Work out the finished part from the listing and answer in its coordinate system (mm). Face numbers are marked on the shaded views. A direction names the side the tool comes from. Coordinates: 2 decimals unless noted, no trailing zeros. Order: outer loops, then holes, each group sorted by start corner. A loop starts at its lowest first (then second) coordinate and runs counter-clockwise, first axis right, second up. Notation, with made-up numbers: M -12,88.5 L 42,88.5 A21 cw 42,93.5 Z; hole C -2,-12 d3. An arc over 180 degrees is marked long. Use a Markdown table: item, result.
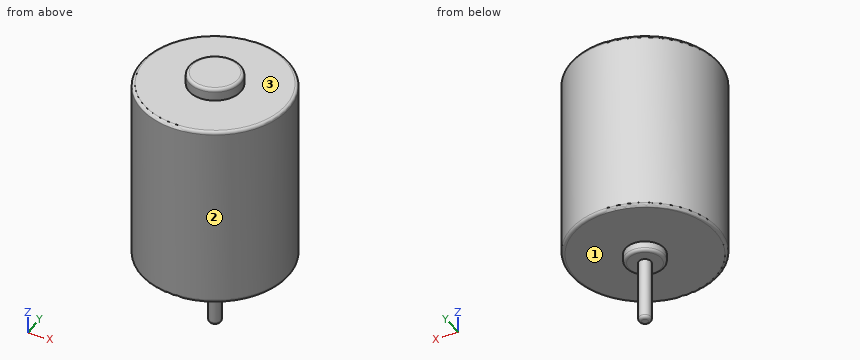
from build123d import *

# Parameters (mm, degrees)
SKETCH1_R           = 12.1
SKETCH1_R_2         = 3.175
SKETCH1_R_3         = 1
BOSS_EXTRUDE1_DEPTH = 30.5
SKETCH1_3_R         = 1
BOSS_EXTRUDE2_DEPTH = 12
SKETCH1_4_R         = 3.175
SKETCH1_4_R_2       = 1
BOSS_EXTRUDE3_DEPTH = 1.6
SKETCH2_R           = 4.25
BOSS_EXTRUDE4_DEPTH = 2
FILLET1_R           = 0.5


with BuildPart() as part:
    # Sketch1 → Boss-Extrude1 (new body)
    # profile 1 of 3: a face of its own
    with BuildSketch(Plane.XY):
        with Locations(Location((0, 0, 0), (0, 0, 180))):
            Circle(SKETCH1_R)
        Circle(SKETCH1_R_2, mode=Mode.SUBTRACT)
    # profile 2 of 3: a face of its own
    with BuildSketch(Plane.XY):
        Circle(SKETCH1_R_2)
        Circle(SKETCH1_R_3, mode=Mode.SUBTRACT)
    # profile 3 of 3: a face of its own
    with BuildSketch(Plane.XY):
        Circle(SKETCH1_R_3)
    extrude(amount=BOSS_EXTRUDE1_DEPTH)

    # Sketch1_3 → Boss-Extrude2 (add)
    with BuildSketch(Plane.XY):
        Circle(SKETCH1_3_R)
    extrude(amount=-BOSS_EXTRUDE2_DEPTH)

    # Sketch1_4 → Boss-Extrude3 (add)
    with BuildSketch(Plane.XY):
        Circle(SKETCH1_4_R)
        Circle(SKETCH1_4_R_2, mode=Mode.SUBTRACT)
    extrude(amount=-BOSS_EXTRUDE3_DEPTH)

    # Sketch2 → Boss-Extrude4 (add)
    with BuildSketch(Plane.XY.offset(30.5)):
        Circle(SKETCH2_R)
    extrude(amount=BOSS_EXTRUDE4_DEPTH)

    # Fillet1
    fillet1_edges = [part.edges().sort_by_distance(p)[0] for p in [
        (-3.175, 0, -1.6),
        (-4.25, 0, 32.5),
        (12.1, 0, 0),
        (12.1, 0, 30.5),
        (-1, 0, -12),
    ]]
    fillet(fillet1_edges, radius=FILLET1_R)


solid = part.part
1. For the marked faces 1, 2 and 3, determine the directions among +Z, -Z, +X, -X, +Y, -Y from which every point of the face is accessible in a straight line to the end or side of a thin tool.
Answers below:
| item | result |
|---|---|
| face 1 | -Z |
| face 2 | +Z, -Z |
| face 3 | +Z |
2. Section A-A on z = 29 is taken. Determine the outline of the cut face in (x, y).
Answers below:
| item | result |
|---|---|
| outline | C 0,0 d24.2 |
3. Flat-ended cylindrical pins translate along their axes: P1, Ø6, axis at x = 7.5, y = -3, coming from the -Z side; P2, Ø5, axis at y = -8, z = 2, coming from the +X side; P3, Ø4, axis at x = -9, z = 9.5, coming from the +Y side. Find the tip coordinate at first contact, or state that the pin passes through.
Answers below:
| item | result |
|---|---|
| P1 | z = 0 |
| P2 | x = 10.78 |
| P3 | y = 9.87 |
4. Find the intervals of material crossed by probe 1 along X at (y, z) = (-0.5, 4); probe 2 along Z at (x, y) = (3.75, -8); probe 3 along X at (y, z) = (9.25, 19.5), in increasing order.
Answers below:
| item | result |
|---|---|
| probe 1 | -12.09 to 12.09 |
| probe 2 | 0 to 30.5 |
| probe 3 | -7.8 to 7.8 |
